```python
from build123d import *

# Parameters (mm, degrees)
ESQUISSE1_W           = 0.875
ESQUISSE1_H           = 1.7
CONG_1_R              = 0.3
ESQUISSE3_R           = 0.275
CONG_1_OF_SYM_TRIE1_R = 0.3
ESQUISSE4_W           = 0.01
ESQUISSE4_H           = 0.8


with BuildPart() as part:
    # Esquisse1 → Révolution1 (revolve)
    with BuildSketch(Plane.XY, mode=Mode.PRIVATE) as r_volution1_sk:
        with Locations((0.4375, 0.85)):
            Rectangle(ESQUISSE1_W, ESQUISSE1_H)
    r_volution1 = revolve(r_volution1_sk.sketch.rotate(Axis((0, 1.7, 0), (0, -1, 0)), 180), axis=Axis((0, 1.7, 0), (0, -1, 0)))

    # Congé1
    cong_1_edges = [part.edges().sort_by_distance(p)[0] for p in [
        (0.875, 1.7, 0),
    ]]
    fillet(cong_1_edges, radius=CONG_1_R)

    # Balayage1: sweep along a path in Esquisse2
    with BuildLine(Plane.XY) as balayage1_path:
        Line((0, 1.7), (0, 3.01))
        ThreePointArc((0, 3.01), (0.234314575, 3.575685425), (0.8, 3.81))
        Line((0.8, 3.81), (4.475, 3.81))
    # Esquisse3 → Balayage1 (sweep)
    with BuildSketch(Plane(origin=(0, 1.7, 0), x_dir=(1, 0, 0), z_dir=(0, 1, 0))):
        Circle(ESQUISSE3_R)
    balayage1 = sweep(path=balayage1_path.line)


with BuildPart() as sym_trie1_1:
    # Symétrie1: Révolution1, Balayage1 across Top Plane
    add(r_volution1.mirror(Plane(origin=(0, 0, 0), x_dir=(1, 0, 0), z_dir=(0, 1, 0))))
    add(balayage1.mirror(Plane(origin=(0, 0, 0), x_dir=(1, 0, 0), z_dir=(0, 1, 0))))

    # Congé1 of Symétrie1
    cong_1_of_sym_trie1_edges = [sym_trie1_1.edges().sort_by_distance(p)[0] for p in [
        (0.875, -1.7, 0),
    ]]
    fillet(cong_1_of_sym_trie1_edges, radius=CONG_1_OF_SYM_TRIE1_R)


with BuildPart() as part_1:
    add(part.part)

    # Symétrie1 united with what the copies to: union Symétrie1_1
    add(sym_trie1_1.part)

    # Esquisse4 → Enlèvement de matière-Révolution1 (revolve, cut)
    with BuildSketch(Plane.XY):
        with Locations((-0.87, 0.7)):
            Rectangle(ESQUISSE4_W, ESQUISSE4_H)
    revolve(axis=Axis((0, -1.4, 0), (0, 1, 0)), mode=Mode.SUBTRACT)


solid = part_1.part
```
Input: part model. Units: mm. Frame: model coordinates. Round coordinates to 2 decimals unless told otherwise and drop trailing zeros. Write each loop counter-clockwise with the first axis right and the second up, starting at its lowest first coordinate (ties: lowest second). Pieces come first, ordered by that corner, then holes. Notation, with made-up numbers: M -26.5,68 L 14.5,68 A23 cw 14.5,104 Z; hole C -11,72.5 d9. An arc over 180 degrees is marked long. Write each question's results on one line, items separated by ' | '.
Q1. Line query: line 1 along Y through (x, z) = (-0.1, -0.3); line 2 along Z through (x, y) = (0, 2.5) (3 decimals). Output: solid intervals per line, ascending.
Results:
line 1: y = -1.7 to 1.7 | line 2: z = -0.275 to 0.275
Q2. Section query D-D (y = -2.25). Return loops of the section in (x, z) (3 decimals), and give its area (3 significant figures).
Results:
outline: C 0,0 d0.55 | area: 0.238 mm^2
Q3. Pin query (flat end, axial travel): P1, Ø0.9, axis at x = 0.5, z = -0.5, coming from the -Y side; P2, Ø0.9, axis at x = 0, z = 0, coming from the -Y side. Return the tip coordinate at first contact, or that it passes through.
Results:
P1: stops at y = -4.06 | P2: stops at y = -4.03
Q4. Section query C-C (y = -0.25). Return loops of the section in (x, z) (3 decimals), and give its area (3 significant figures).
Results:
outline: C 0,0 d1.75 | area: 2.41 mm^2
Q5. Section query B-B (x = 2.85). Return loops of the section in (y, z) (3 decimals).
Results:
outline: C -3.81,0 d0.55; C 3.81,0 d0.55
